Verification items for this drawing (mm, ordinates from the low corner). A direction names the side the tool comes from. Coordinates: 2 decimals unless noted, no trailing zeros. Order: outer loops, then holes, each group sorted by start corner. A loop starts at its lowest first (then second) coordinate and runs counter-clockwise, first axis right, second up. Notation, with made-up numbers: M 50.5,75 L 80.5,75 A23 ccw 80.5,108 Z; hole C 30.25,-30 d3. An arc over 180 degrees is marked long. One line per item, written item: value. Start each with the question number.
1) Sectioned sample at D-D, the plane x = 47. Enter the section's corners in (y, z).
2) Go/stop test with flat-tipped pins: P1, Ø5, axis at x = 6.5, y = 60, coming from the -Z side; P2, Ø7.5, axis at y = 45, z = 28, coming from the +X side; P3, Ø2, axis at x = 36.5, z = 6, coming from the +Y side; P4, Ø12.5, axis at x = 25.5, y = 11, coming from the +Z side. Record where each tip stops, or that it passes through.
3) Access from +Z, -Z, +X, -X, +Y, -Y to the whole of each face (thin tool, end or side, straight path). Record for the marked faces 5, 6, 7, 8 and 9.
4) Sectioned sample at A-A, the plane x = 35. Enter the section's corners in (y, z), then the cut area to 3 significant figures.
5) Thickness scan on L1, parallel to Z at x = 42.5, y = 50.8; L2, parallel to Y at x = 5.5, z = 32; L3, parallel to X at y = 56, z = 19. Record the ranges inside material, lowest first. Write a range as from..to.
6) Sectioned sample at C-C, the plane y = 50.8. Enter the section's corners in (x, z).
7) Draft check along Z on the marked faces 1, 2, 3 and 4. Enter one of: pulls with the +Z half, pulls with the -Z half, needs draft (parallel to the pull), parting line crosses it, or undercut.
8) Sectioned sample at B-B, the plane z = 25.4. Enter the section's corners in (x, y).
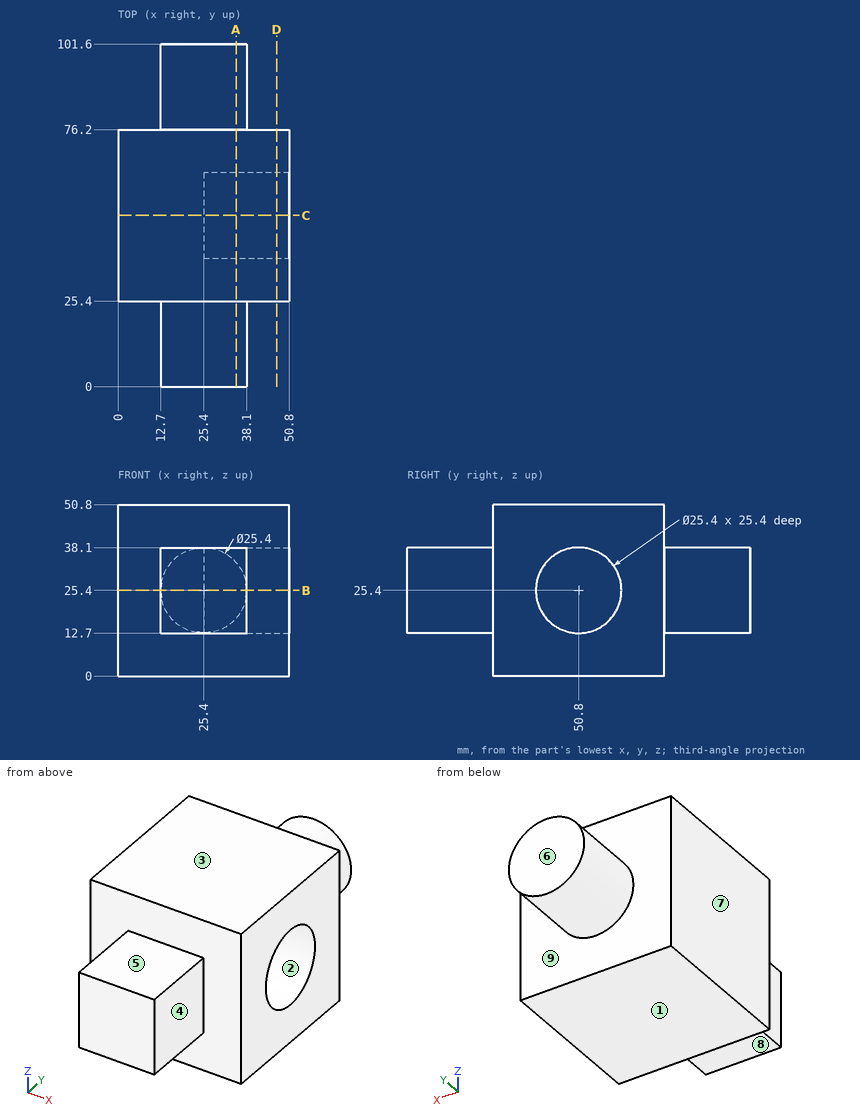
Final values:
1. outline: M 25.4,0 L 76.2,0 L 76.2,50.8 L 25.4,50.8 Z; hole C 50.8,25.4 d25.4
2. P1: stops at z = 0
2. P2: stops at x = 25.4
2. P3: stops at y = 76.2
2. P4: stops at z = 38.1
3. face 5: +Z, +X, -X, -Y
3. face 6: +Z, -Z, +X, -X, +Y
3. face 7: +Z, -Z, -X, +Y, -Y
3. face 8: -Z, +X, -X, -Y
3. face 9: +Y
4. outline: M 0,12.7 L 25.4,12.7 L 25.4,0 L 76.2,0 L 76.2,17.09 L 101.6,17.09 L 101.6,33.71 L 76.2,33.71 L 76.2,50.8 L 25.4,50.8 L 25.4,38.1 L 0,38.1 Z; hole C 50.8,25.4 d25.4
4. area: 3,140 mm^2
5. L1: z = 0..12.7, 38.1..50.8
5. L2: y = 25.4..76.2
5. L3: x = 0..25.4
6. outline: M 0,0 L 50.8,0 L 50.8,12.7 L 25.4,12.7 L 25.4,38.1 L 50.8,38.1 L 50.8,50.8 L 0,50.8 Z
7. face 1: pulls with the -Z half
7. face 2: undercut
7. face 3: pulls with the +Z half
7. face 4: needs draft
8. outline: M 0,25.4 L 12.7,25.4 L 12.7,0 L 38.1,0 L 38.1,25.4 L 50.8,25.4 L 50.8,38.1 L 25.4,38.1 L 25.4,63.5 L 50.8,63.5 L 50.8,76.2 L 38.1,76.2 L 38.1,101.6 L 12.7,101.6 L 12.7,76.2 L 0,76.2 Z
